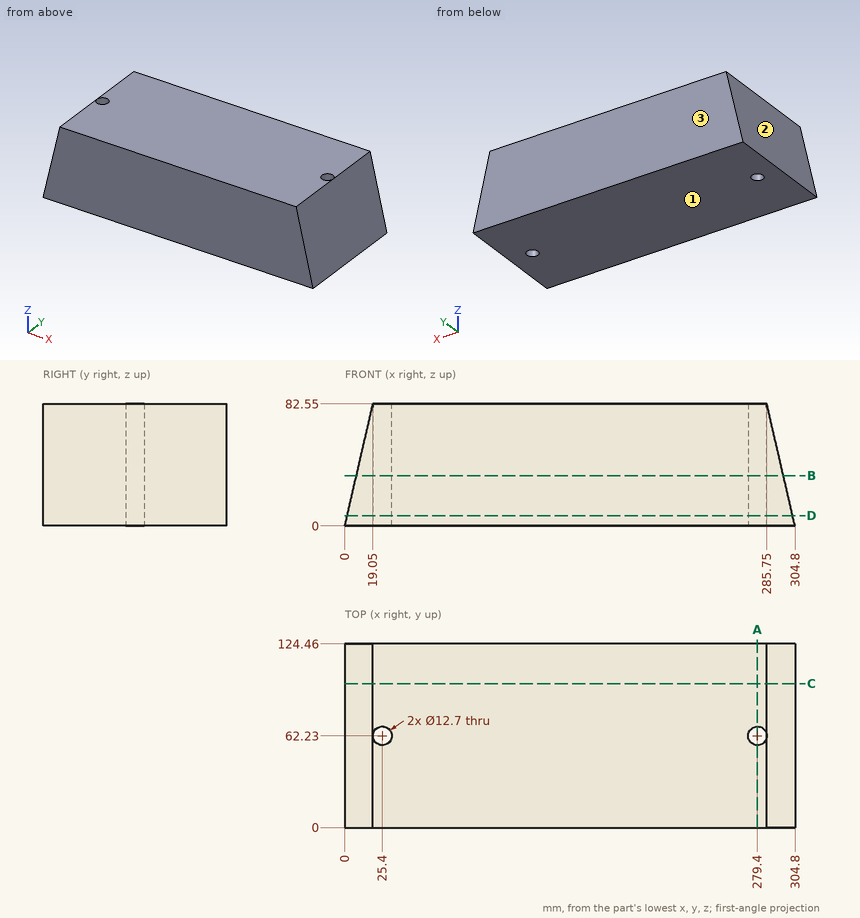
Could you check a few things on this drawing? It's one solid part, dimensions in mm from its lowest x, y, z. Give positions to 0.01 mm unless a question says otherwise; leave off trailing zeros. Write each loop counter-clockwise with the first axis right and the second up, starting at its lowest first coordinate (ties: lowest second). Pieces come first, ordered by that corner, then holes. Notation, with made-up numbers: (78.5, 29.5) - (115.5, 29.5) arc R13 ccw to (115.5, 40.5) - close; hole circle Ø5 at (-23, 37). An arc over 180 degrees is marked (long way). Use CSV: the item, a comma, the result in double quotes. Start each with the question number.
Item 1: I want a section at B-B, the plane z = 34. Please give me the cut outline in (x, y).
Item 2: I want a section at D-D, the plane z = 7. Please give me the cut outline in (x, y), then the cut area to 3 significant figures.
Item 3: If we mould it in two halves opening along Z, with no side actions, what happens to the marked faces 1, 2 and 3? For each: pulls with the +Z half, pulls with the -Z half, needs draft (parallel to the pull), parting line crosses it, or undercut.
Item 4: If I drill on line 1 along Y through (x, z) = (279, 34); line 2 along X through (y, z) = (62, 26); line 3 along X through (y, z) = (59, 72), over which ranges is the centre line in solid material (lowest first)?
Item 5: I'm going to push flat-ended pins straight in: pin 1 (7.5 mm diameter, centred on x = 25.4, y = 62.23, fed in from +Z); pin 2 (4 mm diameter, centred on y = 40, z = 37.5, fed in from +X); pin 3 (20.5 mm diameter, centred on x = 279.4, y = 62.23, fed in from +Z); pin 4 (1.5 mm diameter, centred on y = 19.5, z = 8.5, fed in from -X). Where does each tip first touch, or does it pass through?
Item 6: I want a section at A-A, the plane x = 279.4. Please give me the cut outline in (y, z), then the cut area to 3 significant figures.
Item 7: I want a section at C-C, the plane y = 97.5. Please give me the cut outline in (x, z), then the cut area to 3 significant figures.
Findings:
1,outline,"(7.85, 0) - (296.95, 0) - (296.95, 124.46) - (7.85, 124.46) - close; hole circle Ø12.7 at (25.4, 62.23); hole circle Ø12.7 at (279.4, 62.23)"
2,outline,"(1.62, 0) - (303.18, 0) - (303.18, 124.46) - (1.62, 124.46) - close; hole circle Ø12.7 at (25.4, 62.23); hole circle Ø12.7 at (279.4, 62.23)"
2,area,"37,300 mm2"
3,face 1,"pulls with the -Z half"
3,face 2,"pulls with the +Z half"
3,face 3,"needs draft"
4,line 1,"y = 0 to 55.89, 68.57 to 124.46"
4,line 2,"x = 6 to 19.05, 31.75 to 273.05, 285.75 to 298.8"
4,line 3,"x = 16.62 to 19.93, 30.87 to 273.93, 284.87 to 288.18"
5,pin 1,"passes through"
5,pin 2,"stops at x = 296.61"
5,pin 3,"stops at z = 82.55"
5,pin 4,"stops at x = 1.79"
6,outline,"(0, 0) - (55.88, 0) - (55.88, 82.55) - (0, 82.55) - close; (68.58, 0) - (124.46, 0) - (124.46, 82.55) - (68.58, 82.55) - close"
6,area,"9,230 mm2"
7,outline,"(0, 0) - (304.8, 0) - (285.75, 82.55) - (19.05, 82.55) - close"
7,area,"23,600 mm2"
